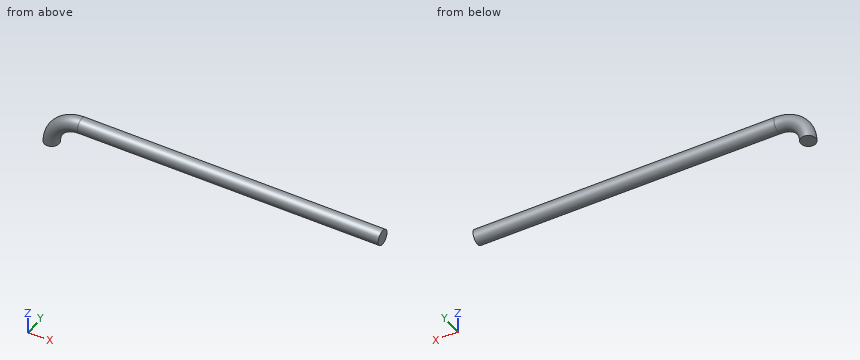
from build123d import *

# Parameters (mm, degrees)
TORUS_R                = 0.25
TORUS_ANGLE            = 90
CYLINDER_R             = 0.25
CYLINDER_DEPTH         = 10
FUSION_PITCH_ANGLE     = -90
FUSION_PLACEMENT_ANGLE = 90


with BuildPart() as torus:
    # Torus → Torus (revolve)
    with BuildSketch(Plane.XZ):
        with Locations((1, 0)):
            Circle(TORUS_R)
    revolve(axis=Axis((0, 0, 0), (0, 0, 1)), revolution_arc=TORUS_ANGLE)


with BuildPart() as fusion:
    # Cylinder → Cylinder (new body)
    with BuildSketch(Plane(origin=(1, 0, 0), x_dir=(1, 0, 0), z_dir=(0, -1, 0))):
        Circle(CYLINDER_R)
    extrude(amount=CYLINDER_DEPTH)

    # Fusion: union Torus
    add(torus.part)


with BuildPart() as fusion_1:
    # Fusion pitch: moved
    add(fusion.part.rotate(Axis((0, 0, 0), (0, 1, 0)), FUSION_PITCH_ANGLE))


with BuildPart() as fusion_2:
    # Fusion placement: moved
    add(fusion_1.part.moved(Location((31, 0, 0))).rotate(Axis((31, 0, 0), (0, 0, 1)), FUSION_PLACEMENT_ANGLE))


solid = fusion_2.part
The listing builds one solid part. Answer for the finished solid, in the listing's coordinates (mm). Give positions to 0.01 mm unless a question says otherwise; leave off trailing zeros. Write each loop counter-clockwise with the first axis right and the second up, starting at its lowest first coordinate (ties: lowest second). Pieces come first, ordered by that corner, then holes. Notation, with made-up numbers: (18, 52.5) - (37, 52.5) arc R26 ccw to (37, 87.5) - close; hole circle Ø7 at (10, 35). An arc over 180 degrees is marked (long way). Use a Markdown table: item, result.
1. Find the intervals of material crossed by probe 1 along Z at (x, y) = (37.5, 0); probe 2 along X at (y, z) = (0.1, 0.4); probe 3 along Y at (x, z) = (36.75, 0.9), in increasing order. Write a range as from..to.
Values follow:
| item | result |
|---|---|
| probe 1 | z = 0.75..1.25 |
| probe 2 | x = 29.84..30.34 |
| probe 3 | y = -0.23..0.23 |
2. Section B-B on x = 32.5 is taken. Write down the section's boundary in (y, z), plus the area to 3 significant figures.
Values follow:
| item | result |
|---|---|
| outline | circle Ø0.5 at (0, 1) |
| area | 0.196 mm² |
3. Section A-A on y = 0 is taken. Write down the section's boundary in (x, z).
Values follow:
| item | result |
|---|---|
| outline | (29.75, 0) - (30.25, 0) arc R0.75 cw to (31, 0.75) - (41, 0.75) - (41, 1.25) - (31, 1.25) arc R1.25 ccw to start |
